Geometry: final body of the model. Coordinates: model frame, mm. Give positions to 0.01 mm unless a question says otherwise; leave off trailing zeros. Write each loop counter-clockwise with the first axis right and the second up, starting at its lowest first coordinate (ties: lowest second). Pieces come first, ordered by that corner, then holes. Notation, with made-up numbers: M 89.5,75.5 L 117.5,75.5 A17 ccw 117.5,99.5 Z; hole C 33,27 d9. An arc over 180 degrees is marked long. Use a Markdown table: item, result. Add a question column.
(1) Material intervals for L1, parallel to Y at x = 0, z = 36.5; L2, parallel to Y at x = -3.5, z = 21.5; L3, parallel to X at y = 31, z = 5.5, sorted ascending.
(2) Pin query (flat end, axial travel): pin 1 Ø8 at (y, z) = (43.5, 19.5) entering from -X; pin 2 Ø6 at (y, z) = (90, 30) entering from +X; pin 3 Ø8 at (y, z) = (-17.5, 16.5) entering from +X. Return the tip coordinate at first contact, or that it passes through.
(3) Cut plane D-D (x = 125). Output: boundary loops of the cut face in (y, z).
(4) Cut plane B-B (z = 21.5). Output: boundary loops of the cut face in (x, y).
(5) Cut plane C-C (y = 101). Output: boundary loops of the cut face in (x, z), plus the area to 3 significant figures.
(6) Draft query along X for faces 1 (the cylindrical face through (-2.6, 57.38, 24.72)), 2 (the flat face through (-3, 70, 0)), 3 (the flat face through (-163.1, -56, 47.5)). Return one class per face: released by +X, released by -X, zero draft, split by the parting line, or undercut.
(7) Cut plane A-A (x = 0). Output: boundary loops of the cut face in (y, z).
```python
from build123d import *

# Parameters (mm, degrees)
F0_R     = 20
F1_DEPTH = 50
F2_SIZE  = 80
F3_R     = 5
F4_SIZE  = 5


with BuildPart() as f1:
    # F0 (on Top) → F1 (new body)
    with BuildSketch(Plane.XY):
        Polygon((0, 297.3580189822), (-225, -92.3534127208), (225, -92.3534127208), align=None)
        with Locations((0, 37.5503978469)):
            Circle(F0_R, mode=Mode.SUBTRACT)
    extrude(amount=F1_DEPTH)

    # F2
    f2_edges = [f1.edges().sort_by_distance(p)[0] for p in [
        (225, -92.353413, 25),
        (-225, -92.353413, 25),
        (0, 297.358019, 25),
    ]]
    chamfer(f2_edges, length=F2_SIZE)

    # F3
    f3_edges = [f1.edges().sort_by_distance(p)[0] for p in [
        (-20, 37.550398, 50),
        (-20, 37.550398, 0),
    ]]
    fillet(f3_edges, radius=F3_R)

    # F4
    f4_edges = [f1.edges().sort_by_distance(p)[0] for p in [
        (112.5, 102.502303, 50),
        (165, -57.712397, 50),
        (0, -92.353413, 50),
        (-165, -57.712397, 50),
        (-112.5, 102.502303, 50),
        (165, -57.712397, 0),
        (0, -92.353413, 0),
        (112.5, 102.502303, 0),
        (-165, -57.712397, 0),
        (-112.5, 102.502303, 0),
        (0, 228.075987, 0),
        (0, 228.075987, 50),
    ]]
    chamfer(f4_edges, length=F4_SIZE)


solid = f1.part
```
Answer list:
| question | item | result |
|---|---|---|
| 1 | L1 | -92.35 to 17.55, 57.55 to 228.08 |
| 1 | L2 | -92.35 to 17.86, 57.24 to 228.08 |
| 1 | L3 | -153.78 to -18.9, 18.9 to 153.78 |
| 2 | pin 1 | x = -148.87 |
| 2 | pin 2 | x = 121.45 |
| 2 | pin 3 | x = 184.09 |
| 3 | outline | M -92.35,5 L -87.35,0 L 70.85,0 L 80.85,5 L 80.85,45 L 70.85,50 L -87.35,50 L -92.35,45 Z |
| 4 | outline | M -185,-23.07 L -145,-92.35 L 145,-92.35 L 185,-23.07 L 40,228.08 L -40,228.08 Z; hole C 0,37.55 d40 |
| 5 | outline | M -113.37,5 L -107.59,0 L 107.59,0 L 113.37,5 L 113.37,45 L 107.59,50 L -107.59,50 L -113.37,45 Z |
| 5 | area | 11,300 mm² |
| 6 | face 1 | undercut |
| 6 | face 2 | zero draft |
| 6 | face 3 | released by -X |
| 7 | outline | M -92.35,5 L -87.35,0 L 12.55,0 A5 ccw 17.55,5 L 17.55,45 A5 ccw 12.55,50 L -87.35,50 L -92.35,45 Z; M 57.55,5 A5 ccw 62.55,0 L 223.08,0 L 228.08,5 L 228.08,45 L 223.08,50 L 62.55,50 A5 ccw 57.55,45 Z |
